```python
from build123d import *

# Parameters (mm, degrees)
SKETCH2_W           = 34
SKETCH2_H           = 28
BOSS_EXTRUDE1_DEPTH = 20
CUT_EXTRUDE1_DEPTH  = 18
SKETCH4_W           = 31
SKETCH4_H           = 18
CUT_EXTRUDE2_DEPTH  = 9
CUT_EXTRUDE3_REACH  = 38.946
SKETCH5_R           = 3
SKETCH8_W           = 12.6
SKETCH8_H           = 8
CUT_EXTRUDE5_DEPTH  = 8.5
SKETCH11_W          = 20.6
SKETCH11_H          = 8
CUT_EXTRUDE6_DEPTH  = 4.5


with BuildPart() as part:
    # Sketch2 → Boss-Extrude1 (new body)
    with BuildSketch(Plane(origin=(0, 0, 0), x_dir=(1, 0, 0), z_dir=(0, 1, 0))):
        Rectangle(SKETCH2_W, SKETCH2_H)
    extrude(amount=BOSS_EXTRUDE1_DEPTH)

    # Sketch3 → Cut-Extrude1 (cut)
    with BuildSketch(Plane(origin=(0, 20, 0), x_dir=(1, 0, 0), z_dir=(0, 1, 0))):
        with BuildLine():
            Line((-12.5, 6), (-12.5, 5))
            ThreePointArc((-12.5, 5), (-15.5, 2), (-12.5, -1))
            Line((-12.5, -1), (-12.5, -12))
            Line((-12.5, -12), (12.5, -12))
            Line((12.5, -12), (12.5, -1))
            ThreePointArc((12.5, -1), (15.5, 2), (12.5, 5))
            Line((12.5, 5), (12.5, 6))
            Line((12.5, 6), (-12.5, 6))
        make_face()
    extrude(amount=-CUT_EXTRUDE1_DEPTH, mode=Mode.SUBTRACT)

    # Sketch4 → Cut-Extrude2 (cut)
    with BuildSketch(Plane(origin=(0, 20, 0), x_dir=(1, 0, 0), z_dir=(0, 1, 0))):
        with Locations((0, -3)):
            Rectangle(SKETCH4_W, SKETCH4_H)
    extrude(amount=-CUT_EXTRUDE2_DEPTH, mode=Mode.SUBTRACT)

    # Cut-Extrude3: up to this face of the body (flat: up to its plane)
    cut_extrude3_end = Plane(part.part.faces().sort_by_distance((0, 11.482142857, -6))[0])
    # Sketch5 → Cut-Extrude3 (cut, up to the picked face)
    with BuildSketch(Plane(origin=(0, 0, 12), x_dir=(-1, 0, 0), z_dir=(0, 0, -1)), mode=Mode.PRIVATE) as cut_extrude3_sk1:
        with Locations((12.5, 11)):
            Circle(SKETCH5_R)
    cut_extrude3_tool1 = split(extrude(cut_extrude3_sk1.sketch, amount=CUT_EXTRUDE3_REACH, mode=Mode.PRIVATE), bisect_by=cut_extrude3_end, keep=Keep.BOTH, mode=Mode.PRIVATE)
    # Sketch5 → Cut-Extrude3 (cut, up to the picked face)
    with BuildSketch(Plane(origin=(0, 0, 12), x_dir=(-1, 0, 0), z_dir=(0, 0, -1)), mode=Mode.PRIVATE) as cut_extrude3_sk2:
        with Locations((-12.5, 11)):
            Circle(SKETCH5_R)
    cut_extrude3_tool2 = split(extrude(cut_extrude3_sk2.sketch, amount=CUT_EXTRUDE3_REACH, mode=Mode.PRIVATE), bisect_by=cut_extrude3_end, keep=Keep.BOTH, mode=Mode.PRIVATE)
    add(cut_extrude3_tool1.solids().sort_by(Axis((-12.5, 11, 12), (0, 0, -1)))[0], mode=Mode.SUBTRACT)
    add(cut_extrude3_tool2.solids().sort_by(Axis((12.5, 11, 12), (0, 0, -1)))[0], mode=Mode.SUBTRACT)

    # Sketch8 → Cut-Extrude5 (cut)
    with BuildSketch(Plane(origin=(0, 20, 0), x_dir=(1, 0, 0), z_dir=(0, 1, 0))):
        with Locations((0, 10)):
            Rectangle(SKETCH8_W, SKETCH8_H)
    extrude(amount=-CUT_EXTRUDE5_DEPTH, mode=Mode.SUBTRACT)

    # Sketch10 → Cut-Revolve1 (revolve, cut)
    with BuildSketch(Plane(origin=(-6.3, 0, 0), x_dir=(0, 0, -1), z_dir=(1, 0, 0))):
        Polygon((6, 15.5), (14, 15.5), (14, 19.5), (8.5, 19.5), (8.5, 17.5), (6, 17.5), align=None)
    cut_revolve1 = revolve(axis=Axis((-6.3, 15.5, -6), (0, 0, -1)), mode=Mode.SUBTRACT)

    # Mirror1: Cut-Revolve1 across plane
    add(cut_revolve1.mirror(Plane(origin=(0, 0, 0), x_dir=(0, 0, 1), z_dir=(1, 0, 0))), mode=Mode.SUBTRACT)

    # Sketch11 → Cut-Extrude6 (cut)
    with BuildSketch(Plane(origin=(0, 20, 0), x_dir=(1, 0, 0), z_dir=(0, 1, 0))):
        with Locations((0, 10)):
            Rectangle(SKETCH11_W, SKETCH11_H)
    extrude(amount=-CUT_EXTRUDE6_DEPTH, mode=Mode.SUBTRACT)


solid = part.part
```
Here's how the part is built. I have some questions about the finished solid (model axes, mm). A direction names the side the tool comes from. Give positions to 0.01 mm unless a question says otherwise; leave off trailing zeros. Loops run counter-clockwise (first coordinate to the right, second up) from the corner with the lowest first, then second, coordinate; pieces in that order, holes last. Notation, with made-up numbers: M 6.5,-34 L 62.5,-34 A21 ccw 62.5,-7 Z; hole C -27.5,-22.75 d10. An arc over 180 degrees is marked long. Put each result on its own line as item: value. Start each with the question number.
(1) I want a section at C-C on y = 18.5. Please give me the cut outline in (x, z).
(2) I want a section at A-A on z = -9.25. Please give me the cut outline in (x, y).
(3) I want a section at D-D on z = 2. Please give me the cut outline in (x, y), then the cut area to 3 significant figures.
(4) Will these pins go through, and if not, where does the flat tip stop? pin 1 Ø0.6 at (x, z) = (-9, -7) entering from +Y; pin 2 Ø1 at (x, z) = (5.5, 1) entering from -Y; pin 3 Ø4 at (x, z) = (2.5, 6.5) entering from +Y; pin 4 Ø2.5 at (x, z) = (0, -8) entering from +Y.
(5) I want a section at B-B on y = 6.25. Please give me the cut outline in (x, z), then the cut area to 3 significant figures.
(6) If we mould it in two halves opening along X, with no side actions, what happens to faces 4 (the flat face through (0, 10, 14)), 5 (the flat face through (17, 10, 0)), 6 (the flat face through (-12.5, 5, 6)), 7 (the flat face through (-17, 10, 0))? For each: +X half, -X half, draft (parallel to the pull), parting line (faces both ways), or undercut.
(7) For faces 1 (the flat face through (0, 8, -14)), 2 (the cylindrical face through (-7.7, 14.07, -7.23)), 3 (the flat face through (-15.5, 16, 3)), which set-ups out of +Z, -Z, +X, -X, +Y, -Y let a thin tool reach every point of the face, with its end or its side?
(8) I need wall thicknesses on line 1 along Z through (x, y) = (4.5, 4.5); line 2 along X through (y, z) = (14, 2); line 3 along X through (y, z) = (4, 11.75). Which ranges of each line are inside material? Lowest first, please. Write a range as [from, to].
Answer block:
1. outline: M -17,-14 L -10.3,-14 L -10.3,-6 L -15.5,-6 L -15.5,12 L 15.5,12 L 15.5,-6 L 10.3,-6 L 10.3,-14 L 17,-14 L 17,14 L -17,14 Z
2. outline: M -17,0 L 17,0 L 17,20 L 10.3,20 L 10.3,15.5 A4 cw 6.3,11.5 L -6.3,11.5 A4 cw -10.3,15.5 L -10.3,20 L -17,20 Z
3. outline: M -17,0 L 17,0 L 17,20 L 15.5,20 L 15.5,11 A3 cw 12.5,8 L 12.5,2 L -12.5,2 L -12.5,8 A3 cw -15.5,11 L -15.5,20 L -17,20 Z
3. area: 162 mm^2
4. pin 1: y = 15.5
4. pin 2: y = 0
4. pin 3: y = 2
4. pin 4: y = 11.5
5. outline: M -17,-14 L 17,-14 L 17,14 L -17,14 Z; hole M -12.5,-6 L 12.5,-6 L 12.5,-5 A3 ccw 12.5,1 L 12.5,12 L -12.5,12 L -12.5,1 A3 ccw -12.5,-5 Z
5. area: 474 mm^2
6. face 4: draft
6. face 5: +X half
6. face 6: undercut
6. face 7: -X half
7. face 1: -Z, +X, -X, +Y, -Y
7. face 2: -Z, +Y
7. face 3: +Y
8. line 1: [-14, -6], [12, 14]
8. line 2: [-17, -15.5], [15.5, 17]
8. line 3: [-17, -12.5], [12.5, 17]
